from build123d import *

# Parameters (mm, degrees)
BOSS_EXTRUDE1_DEPTH = 12.7
SKETCH3_R           = 2
CUT_EXTRUDE1_DEPTH  = 33.328922036
SKETCH2_R           = 2
CUT_EXTRUDE2_DEPTH  = 32.108519733


with BuildPart() as part:
    # Sketch1 → Boss-Extrude1 (new body)
    with BuildSketch(Plane.XY):
        Polygon((0, 0), (0, 2.54), (25.4, 2.54), (25.4, 12.7), (27.94, 12.7), (27.94, 0), align=None)
    extrude(amount=BOSS_EXTRUDE1_DEPTH)

    # Sketch3 → Cut-Extrude1 (cut, through all)
    with BuildSketch(Plane(origin=(0, 2.54, 0), x_dir=(1, 0, 0), z_dir=(0, 1, 0))):
        with Locations(Location((5.08, -6.35, 0), (0, 0, 270))):
            Circle(SKETCH3_R)
        with Locations(Location((12.7, -6.35, 0), (0, 0, 270))):
            Circle(SKETCH3_R)
    extrude(amount=-CUT_EXTRUDE1_DEPTH, mode=Mode.SUBTRACT)

    # Sketch2 → Cut-Extrude2 (cut, through all)
    with BuildSketch(Plane.ZY.offset(-25.4)):
        with Locations((6.35, 8.89)):
            Circle(SKETCH2_R)
    extrude(amount=-CUT_EXTRUDE2_DEPTH, mode=Mode.SUBTRACT)


solid = part.part
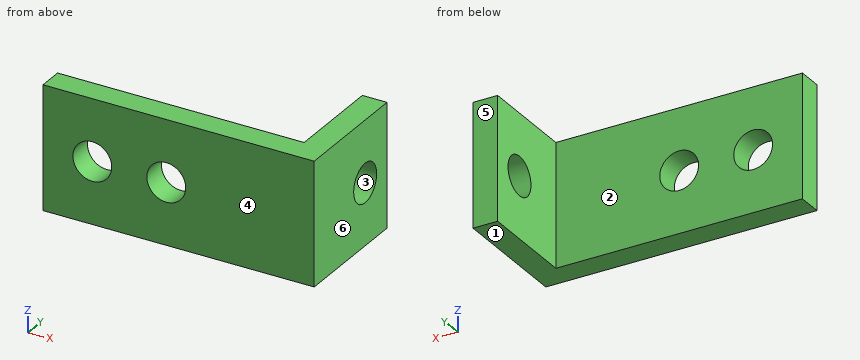
Can you work these out from the model? Positions are in its coordinate system, mm. Face numbers are marked on the shaded views. A direction names the side the tool comes from. Give positions to 0.01 mm unless a question says otherwise; leave off trailing zeros. Order: outer loops, then holes, each group sorted by start corner. A loop starts at its lowest first (then second) coordinate and runs counter-clockwise, first axis right, second up. Notation, with made-up numbers: M 53.25,-35 L 89.25,-35 A22 cw 89.25,-23 Z; hole C 43,27 d7. An arc over 180 degrees is marked long. Use one line per item in the form item = value.
Item 1: For the marked faces 1 and 2, which set-ups out of +Z, -Z, +X, -X, +Y, -Y let a thin tool reach every point of the face, with its end or its side?
Values follow:
face_1 = -Z, +X, -X, +Y, -Y
face_2 = +Z, -Z, -X, +Y
Item 2: If we section it at C-C, the plane x = 12.7: Write out the boundary of the cut face in (y, z).
Values follow:
outline = M 0,0 L 2.54,0 L 2.54,4.35 L 0,4.35 Z; M 0,8.35 L 2.54,8.35 L 2.54,12.7 L 0,12.7 Z
Item 3: If we section it at B-B, the plane y = 8.89: Write out the boundary of the cut face in (x, z).
Values follow:
outline = M 25.4,0 L 27.94,0 L 27.94,4.35 L 25.4,4.35 Z; M 25.4,8.35 L 27.94,8.35 L 27.94,12.7 L 25.4,12.7 Z
Item 4: If I drill on line 1 along X through (y, z) = (1.5, 6.35); line 2 along X through (y, z) = (1, 6); line 3 along X through (y, z) = (11.5, 3.25), over which ranges is the centre line in solid material (lowest first)? Write a range as [from, to].
Values follow:
line_1 = [0, 3.08], [7.08, 10.7], [14.7, 27.94]
line_2 = [0, 3.11], [7.05, 10.73], [14.67, 27.94]
line_3 = [25.4, 27.94]
Item 5: Will these pins go through, and if not, where does the flat tip stop? pin 1 Ø5 at (y, z) = (8.5, 11) entering from -X; pin 2 Ø4 at (x, z) = (14.5, 7.5) entering from +Y; pin 3 Ø6.5 at (y, z) = (8.89, 6.35) entering from +X.
Values follow:
pin_1 = 25.4
pin_2 = 2.54
pin_3 = 27.94
Item 6: If we section it at D-D, the plane z = 10: Write out the boundary of the cut face in (x, y), and give its area (3 significant figures).
Values follow:
outline = M 0,0 L 27.94,0 L 27.94,12.7 L 25.4,12.7 L 25.4,2.54 L 0,2.54 Z
area = 96.8 mm^2
Item 7: Thinking about a two-plate mould opening in Y: for the marked faces 3, 4, 5 and 6, which applies, pulls with the +Y half, pulls with the -Y half, needs draft (parallel to the pull), parting line crosses it, or undercut?
Values follow:
face_3 = undercut
face_4 = pulls with the -Y half
face_5 = pulls with the +Y half
face_6 = needs draft
Item 8: If we section it at A-A, the plane z = 6.35: Write out the boundary of the cut face in (x, y).
Values follow:
outline = M 0,0 L 3.08,0 L 3.08,2.54 L 0,2.54 Z; M 7.08,0 L 10.7,0 L 10.7,2.54 L 7.08,2.54 Z; M 14.7,0 L 27.94,0 L 27.94,6.89 L 25.4,6.89 L 25.4,2.54 L 14.7,2.54 Z; M 25.4,10.89 L 27.94,10.89 L 27.94,12.7 L 25.4,12.7 Z
